Geometry: final body of the model. Coordinates: model frame, mm. Face numbers are marked on the shaded views. A direction names the side the tool comes from. Give positions to 0.01 mm unless a question says otherwise; leave off trailing zeros. Write each loop counter-clockwise with the first axis right and the second up, starting at its lowest first coordinate (ties: lowest second). Pieces come first, ordered by that corner, then holes.
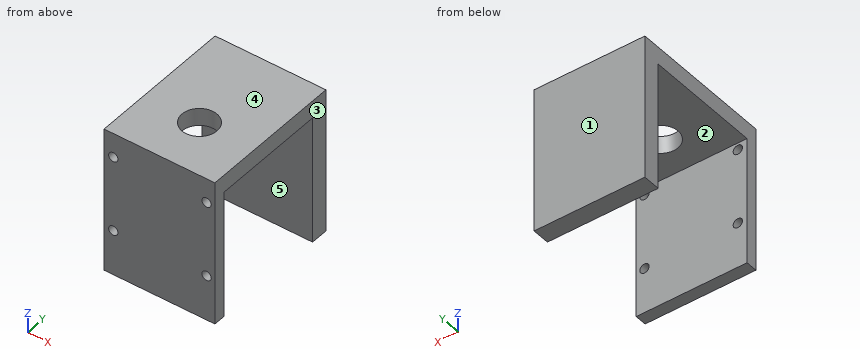
Autodesk Inventor part; units mm, degrees
ref_plane "YZ Plane" through (0, 0, 0) normal (1, 0, 0) x (0, 1, 0)
ref_plane "XZ Plane" through (0, 0, 0) normal (0, 1, 0) x (-1, 0, 0)
ref_plane "XY Plane" through (0, 0, 0) normal (0, 0, 1) x (1, 0, 0)
sketch "スケッチ1" plane through (0, 0, 0) normal (0, 0, 1) x (1, 0, 0)
  line L0 (0, 0) -> (38, 0)
  line L1 (38, 0) -> (38, 24)
  line L2 (38, 24) -> (0, 24)
  line L3 (0, 24) -> (0, 0)
  line L4 (0, 4) -> (38, 4)
  line L5 (13, 33) -> (25, 33)
  line L6 (0, 24) -> (38, 24)
  line L7 (38, 24) -> (38, 44)
  line L8 (38, 44) -> (0, 44)
  line L9 (0, 44) -> (0, 24)
  line L10 (0, 44) -> (38, 44)
  line L11 (38, 44) -> (38, 50)
  line L12 (38, 50) -> (0, 50)
  line L13 (0, 50) -> (0, 44)
  circle A0 centre (19, 33) radius 6
  point P0 (38, 24)
  point P1 (19, 4)
  point P2 (15.6834, 26)
  point P3 (22.3166, 26)
  point P4 (13, 33)
  dimension "d70" = 12
  dimension "d0" = 38
  dimension "d1" = 24
  dimension "d2" = 4
  dimension "d49" = 6
  dimension "d50" = 38
  dimension "d51" = 20
  dimension "d52" = 38
  dimension "d71" = 29
  dimension "d72" = 19
extrude "押し出し1" add sketch "スケッチ1" against normal blind 6 contours L3 L4 L1 L0 | L3 L2 L1 L4 | L9 L8 L7 L2 | L13 L12 L11 L8 | A0 L5 | L5 A0
extrude "押し出し2" add sketch "スケッチ1" against normal blind 50 contours L3 L4 L1 L0 | L13 L12 L11 L8
sketch "スケッチ2" plane through (0, 0, 0) normal (0, 0, 1) x (1, 0, 0)
  line L0 (0, 50) -> (0, 0)
  line L1 (38, 50) -> (0, 50)
  line L2 (38, 0) -> (38, 50)
  line L3 (38, 50) -> (0, 50)
  line L4 (0, 50) -> (0, 0)
  line L5 (0, 0) -> (38, 0)
  point P0 (19, 18)
  point P1 (0, 26)
  point P2 (0, 25)
  point P3 (19, 50)
  point P4 (19, 0)
  point P5 (19, 50)
  dimension "d74" = 32
hole "穴1" at (19, 18, 0) direction (0, 0, -1) diameter 12 depth 8.1 tip angle 118
sketch "スケッチ4" plane through (0, 4, -6) normal (0, 1, 0) x (1, 0, 0)
  point P0 (0, -6)
  point P1 (3.1531, 2.3812)
  point P2 (35.1531, 2.3812)
  point P3 (35.1531, 28.3812)
  point P4 (3.1531, 28.3812)
  dimension "d47" = 32
  dimension "d48" = 26
hole "穴3" at (3.1531, 4, -8.3812) at (35.1531, 4, -8.3812) at (35.1531, 4, -34.3812) at (3.1531, 4, -34.3812) direction (0, -1, 0) diameter 3.2 depth 8.1 tip angle 118
equation "\"d51\" = d1 - d2"
properties part number "ギアボックス2"
Q1. Access query for the marked faces 4 and 5. Directions: +Z, -Z, +X, -X, +Y, -Y. A direction counts if a zero-diameter tool reaches every point of the face in a straight line with its end or side. Return the directions, or none.
Filled sheet:
face 4: +Z, +X, -X, +Y, -Y
face 5: -Z, +X, -X
Q2. Ray query, line 1 along Y through (x, z) = (27, -16); line 2 along Z through (x, y) = (4, 34). Return the intervals inside material, ascending.
Filled sheet:
line 1: y = 0 to 4, 44 to 50
line 2: z = -6 to 0
Q3. Section A-A on z = -43. Output: boundary loops of the cut face in (x, y), plus the area to 3 significant figures.
Filled sheet:
outline: (0, 0) - (38, 0) - (38, 4) - (0, 4) - close; (0, 44) - (38, 44) - (38, 50) - (0, 50) - close
area: 380 mm2
Q4. Section B-B on x = 19. Output: boundary loops of the cut face in (y, z), plus the area to 3 significant figures.
Filled sheet:
outline: (0, -50) - (4, -50) - (4, -6) - (12, -6) - (12, 0) - (0, 0) - close; (24, -6) - (44, -6) - (44, -50) - (50, -50) - (50, 0) - (24, 0) - close
area: 668 mm2
Q5. Section D-D on x = 5.5. Output: boundary loops of the cut face in (y, z).
Filled sheet:
outline: (0, -50) - (4, -50) - (4, -6) - (44, -6) - (44, -50) - (50, -50) - (50, 0) - (0, 0) - close
Q6. Section C-C on y = 18. Output: boundary loops of the cut face in (x, z).
Filled sheet:
outline: (0, -6) - (13, -6) - (13, 0) - (0, 0) - close; (25, -6) - (38, -6) - (38, 0) - (25, 0) - close
Q7. Pin query (flat end, axial travel): P1, Ø3, axis at x = 35.15, z = -34.38, coming from the -Y side; P2, Ø6, axis at x = 4, y = 18, coming from the -Z side. Return the tip coordinate at first contact, or that it passes through.
Filled sheet:
P1: stops at y = 44
P2: stops at z = -6
Q8. Pull-direction query (Y, two-part tool) for the marked faces 1, 2 and 3; classes: released by +Y, released by -Y, zero draft, split by the parting line, or undercut.
Filled sheet:
face 1: released by +Y
face 2: undercut
face 3: zero draft
